CAD build for the part. Positions are in the model's coordinates, mm. A direction names the side the tool comes from. Coordinates: 2 decimals unless noted, no trailing zeros. Order: outer loops, then holes, each group sorted by start corner. A loop starts at its lowest first (then second) coordinate and runs counter-clockwise, first axis right, second up.
from build123d import *

# Parameters (mm, degrees)
EXTRUDE_THIN1_DEPTH        = 82.739
EXTRUDE_THIN1_DEPTH_BACK   = 57.5
CUT_EXTRUDE1_REACH         = 86.901
LPATTERN1_COUNT            = 2
LPATTERN1_PITCH            = 25
LPATTERN1_COL_COUNT        = 2
LPATTERN1_COL_PITCH        = 25
SZKIC1_R                   = 1.6
WYTNIJ_WYCI_GNI_CIE1_DEPTH = 85.901367015


with BuildPart() as part:
    # Sketch1 → Extrude-Thin1 (new, two sides: drawn at the far end of the back side and taken through both)
    with BuildSketch(Plane(origin=(0, 0, 0), x_dir=(0, 0, -1), z_dir=(1, 0, 0)).offset(-EXTRUDE_THIN1_DEPTH_BACK)):
        with BuildLine():
            Line((-17.5, 6.5), (-15.5, 6.5))
            ThreePointArc((-15.5, 6.5), (-14.085786438, 5.914213562), (-13.5, 4.5))
            Line((-13.5, 4.5), (-13.5, 2))
            ThreePointArc((-13.5, 2), (-12.914213562, 0.585786438), (-11.5, 0))
            Line((-11.5, 0), (11.5, 0))
            ThreePointArc((11.5, 0), (12.914213562, 0.585786438), (13.5, 2))
            Line((13.5, 2), (13.5, 4.5))
            ThreePointArc((13.5, 4.5), (14.085786438, 5.914213562), (15.5, 6.5))
            Line((15.5, 6.5), (17.5, 6.5))
            Line((17.5, 6.5), (17.5, 7.5))
            Line((17.5, 7.5), (15.5, 7.5))
            ThreePointArc((15.5, 7.5), (13.378679656, 6.621320344), (12.5, 4.5))
            Line((12.5, 4.5), (12.5, 2))
            ThreePointArc((12.5, 2), (12.207106781, 1.292893219), (11.5, 1))
            Line((11.5, 1), (-11.5, 1))
            ThreePointArc((-11.5, 1), (-12.207106781, 1.292893219), (-12.5, 2))
            Line((-12.5, 2), (-12.5, 4.5))
            ThreePointArc((-12.5, 4.5), (-13.378679656, 6.621320344), (-15.5, 7.5))
            Line((-15.5, 7.5), (-17.5, 7.5))
            Line((-17.5, 7.5), (-17.5, 6.5))
        make_face()
    extrude(amount=EXTRUDE_THIN1_DEPTH + EXTRUDE_THIN1_DEPTH_BACK)

    # Sketch2 → Cut-Extrude1 (cut, up to next)
    with BuildSketch(Plane.XZ, mode=Mode.PRIVATE) as cut_extrude1_sk1:
        with BuildLine():
            Line((-5.875, 3.125), (5.875, 3.125))
            ThreePointArc((5.875, 3.125), (9, 0), (5.875, -3.125))
            Line((5.875, -3.125), (-5.875, -3.125))
            ThreePointArc((-5.875, -3.125), (-9, 0), (-5.875, 3.125))
        make_face()
    cut_extrude1_tool1 = extrude(cut_extrude1_sk1.sketch, amount=-CUT_EXTRUDE1_REACH, mode=Mode.PRIVATE) & part.part
    cut_extrude1 = cut_extrude1_tool1.solids().sort_by_distance((0, 0, 0))[0]
    add(cut_extrude1, mode=Mode.SUBTRACT)

    # LPattern1: Cut-Extrude1 ×2
    with Locations(*[(i * LPATTERN1_PITCH, 0, 0) for i in range(1, LPATTERN1_COUNT)]):
        add(cut_extrude1, mode=Mode.SUBTRACT)

    # LPattern1 col: Cut-Extrude1 ×2
    with Locations(*[(-i * LPATTERN1_COL_PITCH, 0, 0) for i in range(1, LPATTERN1_COL_COUNT)]):
        add(cut_extrude1, mode=Mode.SUBTRACT)

    # Szkic1 → Wytnij-wyciągnięcie1 (cut, through all)
    with BuildSketch(Plane.XZ):
        with Locations(Location((70.2, 0, 0), (0, 0, 270))):
            Circle(SZKIC1_R)
        with Locations(Location((-49.8, 0, 0), (0, 0, 270))):
            Circle(SZKIC1_R)
    extrude(amount=-WYTNIJ_WYCI_GNI_CIE1_DEPTH, mode=Mode.SUBTRACT)


solid = part.part
1) Drill centre lines: probe 1 along Z at (x, y) = (-5.5, 4.5); probe 2 along X at (y, z) = (0.6, 0); probe 3 along Z at (x, y) = (4.5, 7). Where is each one in solid material? Low to high.
2) Pin check, flat tips, straight feed: P1, Ø2, axis at x = 24.5, z = -16.5, coming from the -Y side; P2, Ø3, axis at x = 44, y = 3.5, coming from the -Z side; P3, Ø2, axis at x = 36.5, y = 2, coming from the +Z side; P4, Ø1.9, axis at x = -49.8, z = 0, coming from the -Y side. Stop position of each tip, or through.
3) Slice it at B-B (z = 0). List the corners of the cut face in (x, y).
4) Slice it at C-C (x = 70.2). List the corners of the cut face in (y, z).
5) Which spindle directions (+Z, -Z, +X, -X, +Y, -Y) get a long thin tool onto all of the face, cutting with end or side? Do faces 1 (the cylindrical face through (-16, 0.5, 0.1)), 2 (the flat face through (12, 3, 13.5)), 3 (the flat face through (12, 0, 0)), 4 (the cylindrical face through (11.64, 6.64, -13.4)). Say none if no direction does.
6) Slice it at D-D (z = 7.5). List the corners of the cut face in (x, y), plus the area to 3 significant figures.
7) Slice it at A-A (x = -3.5). List the corners of the cut face in (y, z) (3 decimals).
8) Two-plate mould, pull along Z, no slides. Class faces 5 (the flat face through (12, 3, 12.5)), 6 (the flat face through (82.739, 0.7, 0.1)), 7 (the flat face through (12, 3, -13.5)): released by +Z, released by -Z, zero draft, split by the parting line, or undercut.
Worked out:
1. probe 1: z = -13.5 to -12.5, 12.5 to 13.5
1. probe 2: x = -57.5 to -51.4, -48.2 to -34, -16 to -9, 9 to 16, 34 to 68.6, 71.8 to 82.74
1. probe 3: z = -17.5 to -13.84, 13.84 to 17.5
2. P1: stops at y = 6.5
2. P2: stops at z = -13.56
2. P3: stops at z = 13.5
2. P4: passes through
3. outline: (-57.5, 0) - (-51.4, 0) - (-51.4, 1) - (-57.5, 1) - close; (-48.2, 0) - (-34, 0) - (-34, 1) - (-48.2, 1) - close; (-16, 0) - (-9, 0) - (-9, 1) - (-16, 1) - close; (9, 0) - (16, 0) - (16, 1) - (9, 1) - close; (34, 0) - (68.6, 0) - (68.6, 1) - (34, 1) - close; (71.8, 0) - (82.74, 0) - (82.74, 1) - (71.8, 1) - close
4. outline: (0, -11.5) arc R2 ccw to (2, -13.5) - (4.5, -13.5) arc R2 cw to (6.5, -15.5) - (6.5, -17.5) - (7.5, -17.5) - (7.5, -15.5) arc R3 ccw to (4.5, -12.5) - (2, -12.5) arc R1 cw to (1, -11.5) - (1, -1.6) - (0, -1.6) - close; (0, 1.6) - (1, 1.6) - (1, 11.5) arc R1 cw to (2, 12.5) - (4.5, 12.5) arc R3 ccw to (7.5, 15.5) - (7.5, 17.5) - (6.5, 17.5) - (6.5, 15.5) arc R2 cw to (4.5, 13.5) - (2, 13.5) arc R2 ccw to (0, 11.5) - close
5. face 1: +Y, -Y
5. face 2: +Z, +X, -X, -Y
5. face 3: +Z, -Z, +X, -X, -Y
5. face 4: +X, -X, +Y
6. outline: (-57.5, 0) - (82.74, 0) - (82.74, 1) - (-57.5, 1) - close
6. area: 140 mm2
7. outline: (0, -11.5) arc R2 ccw to (2, -13.5) - (4.5, -13.5) arc R2 cw to (6.5, -15.5) - (6.5, -17.5) - (7.5, -17.5) - (7.5, -15.5) arc R3 ccw to (4.5, -12.5) - (2, -12.5) arc R1 cw to (1, -11.5) - (1, -3.125) - (0, -3.125) - close; (0, 3.125) - (1, 3.125) - (1, 11.5) arc R1 cw to (2, 12.5) - (4.5, 12.5) arc R3 ccw to (7.5, 15.5) - (7.5, 17.5) - (6.5, 17.5) - (6.5, 15.5) arc R2 cw to (4.5, 13.5) - (2, 13.5) arc R2 ccw to (0, 11.5) - close
8. face 5: undercut
8. face 6: zero draft
8. face 7: released by -Z
